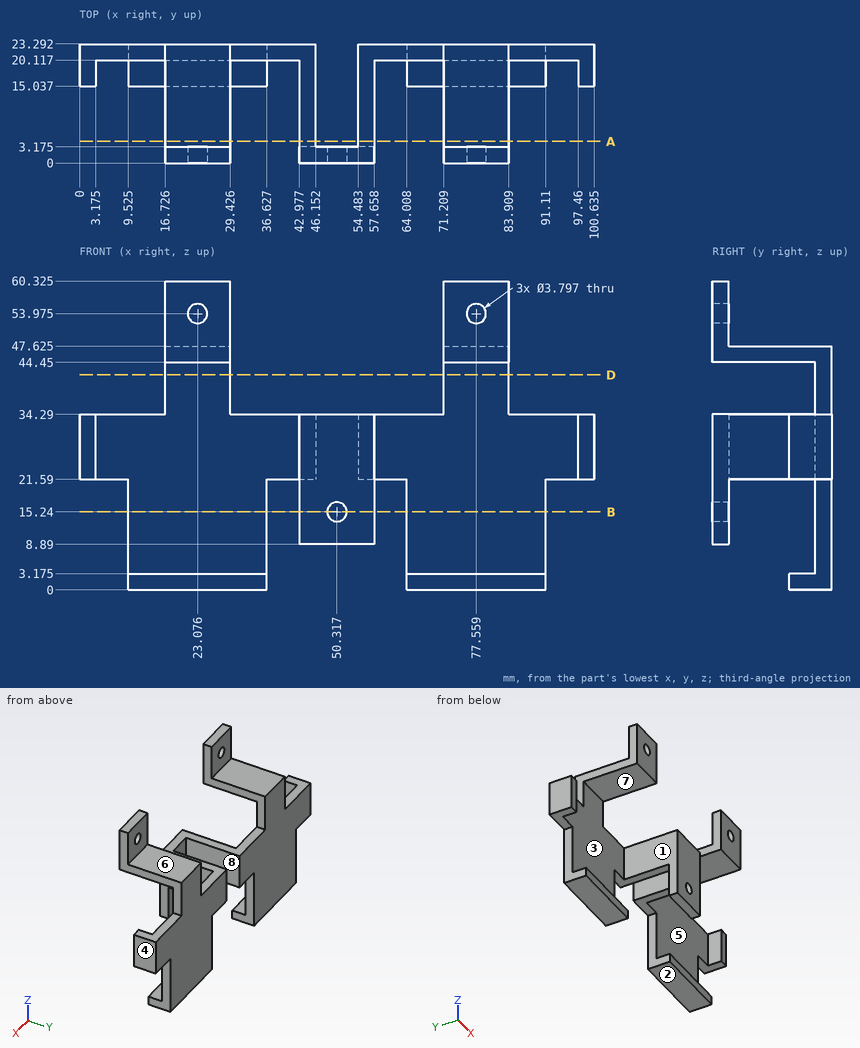
The drawing under review shows one solid part. Ordinate dimensions are in mm from its lowest x, y, z. A direction names the side the tool comes from. Coordinates: 2 decimals unless noted, no trailing zeros. Write each loop counter-clockwise with the first axis right and the second up, starting at its lowest first coordinate (ties: lowest second). Pieces come first, ordered by that corner, then holes. Notation, with made-up numbers: (-28.5, 37.5) -> (8.5, 37.5) arc R21 ccw to (8.5, 68.5) -> close; hole circle Ø2 at (-26.75, -30.5). An arc over 180 degrees is marked (long way). One line per item, written item: value. Start each with the question number.
Q1. Add section A-A, the plane y = 4.25. Count the separate pieces of the cut face and the enclosed holes in it, then the cut area to 3 significant figures.
Q2. For the marked faces 5, 6, 7 and 8, list the 3-axis set-ups (+Z, -Z, +X, -X, +Y, -Y) from which the entire face can be reached by the end or side of a thin tool; tool diameter is ignored.
Q3. The part is to be moulded in two halves that separate along X. For the marked faces 1, 2, 3 and 4, say which applies: +X half, -X half, draft (parallel to the pull), parting line (faces both ways), or undercut.
Q4. To check wall thickness, follow probe 1 along X at (y, z) = (18.5, 32) (1 decimal); probe 2 along X at (y, z) = (1.8, 15.24); probe 3 along X at (y, z) = (3, 53.5) (1 decimal). State the ranges of each line that lie inside material, in increasing order.
Q5. Clearance check with flat-ended pins moving along their axes: P1, Ø5, axis at x = 12.5, y = 3, coming from the +Z side; P2, Ø4, axis at x = 3, y = 20.5, coming from the -Z side; P3, Ø2.5, axis at x = 82.5, y = 16.5, coming from the +Z side (3 decimals); P4, Ø11.5, axis at y = 12.5, z = 44.5, coming from the -X side. State where each tip first meets the part, or that it passes through.
Q6. Add section D-D, the plane z = 42. Give the boundary of the cut face in (x, y).
Q7. Add section B-B, the plane z = 15.24. Give the boundary of the cut face in (x, y) (1 decimal), then the cut area to 3 significant figures.
Response:
1. separate pieces: 4
1. enclosed holes: 0
1. area: 161 mm²
2. face 5: -Y
2. face 6: +Z, +X, -X, +Y
2. face 7: +X, -X, -Y
2. face 8: +Z, -Z, +Y
3. face 1: undercut
3. face 2: draft
3. face 3: undercut
3. face 4: +X half
4. probe 1: 0 to 3.2, 43 to 46.2, 54.5 to 57.7, 97.5 to 100.6
4. probe 2: 42.98 to 48.42, 52.22 to 57.66
4. probe 3: 16.7 to 21.2, 24.9 to 29.4, 71.2 to 75.7, 79.4 to 83.9
5. P1: through
5. P2: z = 21.59
5. P3: z = 47.625
5. P4: x = 16.73
6. outline: (16.73, 20.12) -> (29.43, 20.12) -> (29.43, 23.29) -> (16.73, 23.29) -> close; (71.21, 20.12) -> (83.91, 20.12) -> (83.91, 23.29) -> (71.21, 23.29) -> close
7. outline: (9.5, 20.1) -> (36.6, 20.1) -> (36.6, 23.3) -> (9.5, 23.3) -> close; (43, 0) -> (48.4, 0) -> (48.4, 3.2) -> (43, 3.2) -> close; (52.2, 0) -> (57.7, 0) -> (57.7, 3.2) -> (52.2, 3.2) -> close; (64, 20.1) -> (91.1, 20.1) -> (91.1, 23.3) -> (64, 23.3) -> close
7. area: 207 mm²
